Here's how the part is built. I have some questions about the finished solid (model axes, mm). A direction names the side the tool comes from. Round coordinates to 2 decimals unless told otherwise and drop trailing zeros. Loops run counter-clockwise (first coordinate to the right, second up) from the corner with the lowest first, then second, coordinate; pieces in that order, holes last. Notation, with made-up numbers: (-2, 6.25) -> (21, 6.25) arc R20 cw to (21, 19.25) -> close; hole circle Ø10 at (89, 65). An arc over 180 degrees is marked (long way). Use one line per item in the form item = value. Start each with the question number.
Item 1: If I drill on L1, parallel to Y at x = 35, z = -9; L2, parallel to X at y = 43.5, z = 3.5; L3, parallel to X at y = 97.5, z = -10, over which ranges is the centre line in solid material (lowest first)? Write a range as [from, to].
Item 2: Thinking about a two-plate mould opening in Z: for faces 4 (the face through (59, 11, -2)), 5 (the face through (59, 94.75, -4)), 6 (the face through (5.7, 100, -1)), 7 (the face through (60, 47, 0)), which applies, released by +Z, released by -Z, zero draft, split by the parting line, or undercut?
Item 3: If we section it at B-B (y = 86): Write out the boundary of the cut face in (x, z).
Item 4: If we section it at A-A (x = 34): Write out the boundary of the cut face in (y, z), then the cut area to 3 significant figures.
Item 5: For faces 1 (the face through (31, -3, -3)), 2 (the face through (38, 101, -7)), 3 (the face through (54.75, 99, -4)), which set-ups out of +Z, -Z, +X, -X, +Y, -Y let a thin tool reach every point of the face, with its end or its side?
Item 6: If we section it at C-C (x = 15): Write out the boundary of the cut face in (y, z), then the cut area to 3 significant figures.
Item 7: I'm going to push a flat-ended pin straight in: pin 1 Ø4 at (x, y) = (57, 7) entering from +Z. Where does the tip first touch, or does it pass through?
```python
from build123d import *

# Parameters (mm, degrees)
SKICA1_W                 = 67
SKICA1_H                 = 107
SKICA1_W_2               = 61
SKICA1_H_2               = 101
P_IDAT_VYSUNUT_M1_DEPTH  = 7
P_IDAT_VYSUNUT_M2_DEPTH  = 13
SKICA3_R                 = 1.5
ODEBRAT_VYSUNUT_M1_DEPTH = 13
ODEBRAT_START            = -4.8
ODEBRAT_VYSUNUT_M2_DEPTH = 4.8
ODEBRAT_VYSUNUT_M4_DEPTH = 123.804723036
ZAOBLIT1_R               = 3
SKICA5_W                 = 4
SKICA5_H                 = 8.5
SKICA5_H_2               = 13
P_IDAT_VYSUNUT_M3_DEPTH  = 3
ZKOSEN_1_SIZE            = 3
SKICA6_W                 = 4
SKICA6_H                 = 8.5
SKICA6_H_2               = 13
P_IDAT_VYSUNUT_M4_DEPTH  = 3
ZKOSEN_2_SIZE            = 3
SKICA7_W                 = 9.5
SKICA7_H                 = 7.5
ODEBRAT_VYSUNUT_M3_DEPTH = 10
SKICA9_W                 = 9.5
SKICA9_H                 = 1.25
P_IDAT_VYSUNUT_M5_DEPTH  = 4
ZAOBLIT2_R               = 1
SKICA10_W                = 19.3
SKICA10_H                = 2.8
ODEBRAT_VYSUNUT_M5_DEPTH = 6
SKICA11_R                = 1.5
ODEBRAT_VYSUNUT_M6_DEPTH = 4
SKICA13_R                = 2.5
P_IDAT_VYSUNUT_M6_DEPTH  = 1


with BuildPart() as part:
    # Skica1 → Přidat vysunutím1 (new body)
    with BuildSketch(Plane.XY):
        with Locations((30.5, 50.5)):
            Rectangle(SKICA1_W, SKICA1_H)
        with Locations((30.5, 50.5)):
            Rectangle(SKICA1_W_2, SKICA1_H_2, mode=Mode.SUBTRACT)
    extrude(amount=P_IDAT_VYSUNUT_M1_DEPTH)

    # Skica2 → Přidat vysunutím2 (add)
    with BuildSketch(Plane(origin=(0, 0, 0), x_dir=(-1, 0, 0), z_dir=(0, 0, -1))):
        with BuildLine():
            ThreePointArc((-53, 0), (-53.14730658, -1.5281381), (-53.583801513, -3))
            Line((-53.583801513, -3), (-7.416198487, -3))
            ThreePointArc((-7.416198487, -3), (-7.85269342, -1.5281381), (-8, 0))
            Line((-8, 0), (-53, 0))
        make_face()
        with BuildLine():
            ThreePointArc((-61, 8), (-62.5281381, 7.85269342), (-64, 7.416198487))
            Line((-64, 7.416198487), (-64, -3))
            Line((-64, -3), (-53.583801513, -3))
            ThreePointArc((-53.583801513, -3), (-53.14730658, -1.5281381), (-53, 0))
            Line((-53, 0), (-61, 0))
            Line((-61, 0), (-61, 8))
        make_face()
        with BuildLine():
            ThreePointArc((-53, 0), (-55.343145751, 5.656854249), (-61, 8))
            Line((-61, 8), (-61, 0))
            Line((-61, 0), (-53, 0))
        make_face()
        with BuildLine():
            ThreePointArc((-61, 93), (-62.5281381, 93.14730658), (-64, 93.583801513))
            Line((-64, 93.583801513), (-64, 7.416198487))
            ThreePointArc((-64, 7.416198487), (-62.5281381, 7.85269342), (-61, 8))
            Line((-61, 8), (-61, 93))
        make_face()
        with BuildLine():
            Line((-53.583801513, 104), (-64, 104))
            Line((-64, 104), (-64, 93.583801513))
            ThreePointArc((-64, 93.583801513), (-62.5281381, 93.14730658), (-61, 93))
            Line((-61, 93), (-61, 101))
            Line((-61, 101), (-53, 101))
            ThreePointArc((-53, 101), (-53.14730658, 102.5281381), (-53.583801513, 104))
        make_face()
        with BuildLine():
            ThreePointArc((-61, 93), (-55.343145751, 95.343145751), (-53, 101))
            Line((-53, 101), (-61, 101))
            Line((-61, 101), (-61, 93))
        make_face()
        with BuildLine():
            Line((-7.416198487, 104), (-53.583801513, 104))
            ThreePointArc((-53.583801513, 104), (-53.14730658, 102.5281381), (-53, 101))
            Line((-53, 101), (-8, 101))
            ThreePointArc((-8, 101), (-7.85269342, 102.5281381), (-7.416198487, 104))
        make_face()
        with BuildLine():
            Line((3, 104), (-7.416198487, 104))
            ThreePointArc((-7.416198487, 104), (-7.85269342, 102.5281381), (-8, 101))
            Line((-8, 101), (0, 101))
            Line((0, 101), (0, 93))
            ThreePointArc((0, 93), (1.5281381, 93.14730658), (3, 93.583801513))
            Line((3, 93.583801513), (3, 104))
        make_face()
        with BuildLine():
            Line((0, 101), (-8, 101))
            ThreePointArc((-8, 101), (-5.656854249, 95.343145751), (0, 93))
            Line((0, 93), (0, 101))
        make_face()
        with BuildLine():
            Line((3, 7.416198487), (3, 93.583801513))
            ThreePointArc((3, 93.583801513), (1.5281381, 93.14730658), (0, 93))
            Line((0, 93), (0, 8))
            ThreePointArc((0, 8), (1.5281381, 7.85269342), (3, 7.416198487))
        make_face()
        with BuildLine():
            Line((3, -3), (3, 7.416198487))
            ThreePointArc((3, 7.416198487), (1.5281381, 7.85269342), (0, 8))
            Line((0, 8), (0, 0))
            Line((0, 0), (-8, 0))
            ThreePointArc((-8, 0), (-7.85269342, -1.5281381), (-7.416198487, -3))
            Line((-7.416198487, -3), (3, -3))
        make_face()
        with BuildLine():
            Line((0, 0), (0, 8))
            ThreePointArc((0, 8), (-5.656854249, 5.656854249), (-8, 0))
            Line((-8, 0), (0, 0))
        make_face()
    extrude(amount=P_IDAT_VYSUNUT_M2_DEPTH)

    # Skica3 → Odebrat vysunutím1 (cut)
    with BuildSketch(Plane.XY):
        with Locations((3.5, 97.5)):
            Circle(SKICA3_R)
        with Locations((3.5, 3.5)):
            Circle(SKICA3_R)
        with Locations((57.5, 3.5)):
            Circle(SKICA3_R)
        with Locations((57.5, 97.5)):
            Circle(SKICA3_R)
    extrude(amount=-ODEBRAT_VYSUNUT_M1_DEPTH, mode=Mode.SUBTRACT)

    # Skica4 → Odebrat vysunutím2 (cut)
    with BuildSketch(Plane(origin=(0, 0, -13), x_dir=(-1, 0, 0), z_dir=(0, 0, -1)).offset(ODEBRAT_START)):
        with BuildLine():
            Line((-53, 101), (-61, 101))
            Line((-61, 101), (-61, 93))
            ThreePointArc((-61, 93), (-55.343145751, 95.343145751), (-53, 101))
        make_face()
    extrude(amount=ODEBRAT_VYSUNUT_M2_DEPTH, mode=Mode.SUBTRACT)

    # Skica8 → Odebrat vysunutím4 (cut, through all)
    with BuildSketch(Plane.XY):
        with BuildLine():
            Line((61, 94.75), (57.5, 94.75))
            ThreePointArc((57.5, 94.75), (55.555456352, 95.555456352), (54.75, 97.5))
            Line((54.75, 97.5), (54.75, 101))
            Line((54.75, 101), (53, 101))
            ThreePointArc((53, 101), (55.343145751, 95.343145751), (61, 93))
            Line((61, 93), (61, 94.75))
        make_face()
    extrude(amount=-ODEBRAT_VYSUNUT_M4_DEPTH, mode=Mode.SUBTRACT)

    # Zaoblit1
    zaoblit1_edges = [part.edges().sort_by_distance(p)[0] for p in [
        (-3, 104, -3),
        (64, 104, -3),
        (64, -3, -3),
        (-3, -3, -3),
    ]]
    fillet(zaoblit1_edges, radius=ZAOBLIT1_R)

    # Skica5 → Přidat vysunutím3 (add)
    with BuildSketch(Plane(origin=(0, 0, 0), x_dir=(0, 0, -1), z_dir=(1, 0, 0))):
        with Locations((2, 11.25)):
            Rectangle(SKICA5_W, SKICA5_H)
        with Locations((2, 47.5)):
            Rectangle(SKICA5_W, SKICA5_H_2)
    extrude(amount=P_IDAT_VYSUNUT_M3_DEPTH)

    # Zkosení1
    zkosen_1_edges = [part.edges().sort_by_distance(p)[0] for p in [
        (3, 11.458099244, -4),
        (3, 47.5, -4),
    ]]
    chamfer(zkosen_1_edges, length=ZKOSEN_1_SIZE - 0.0001)  # a hair under: the kernel refuses the full size

    # Skica6 → Přidat vysunutím4 (add)
    with BuildSketch(Plane.ZY.offset(-61)):
        with Locations((-2, 11.25)):
            Rectangle(SKICA6_W, SKICA6_H)
        with Locations((-2, 47.5)):
            Rectangle(SKICA6_W, SKICA6_H_2)
    extrude(amount=P_IDAT_VYSUNUT_M4_DEPTH)

    # Zkosení2
    zkosen_2_edges = [part.edges().sort_by_distance(p)[0] for p in [
        (58, 11.458099244, -4),
        (58, 47.5, -4),
    ]]
    chamfer(zkosen_2_edges, length=ZKOSEN_2_SIZE - 0.0001)  # a hair under: the kernel refuses the full size

    # Skica7 → Odebrat vysunutím3 (cut)
    with BuildSketch(Plane(origin=(0, 104, 0), x_dir=(1, 0, 0), z_dir=(0, 1, 0))):
        with Locations((48.75, 9.25)):
            Rectangle(SKICA7_W, SKICA7_H)
    extrude(amount=-ODEBRAT_VYSUNUT_M3_DEPTH, mode=Mode.SUBTRACT)

    # Skica9 → Přidat vysunutím5 (add)
    with BuildSketch(Plane(origin=(0, 0, -13), x_dir=(-1, 0, 0), z_dir=(0, 0, -1))):
        with Locations((-48.75, 103.375)):
            Rectangle(SKICA9_W, SKICA9_H)
    extrude(amount=-P_IDAT_VYSUNUT_M5_DEPTH)

    # Zaoblit2
    zaoblit2_edges = [part.edges().sort_by_distance(p)[0] for p in [
        (53.5, 103.375, -9),
        (44, 103.375, -9),
    ]]
    fillet(zaoblit2_edges, radius=ZAOBLIT2_R)

    # Skica10 → Odebrat vysunutím5 (cut, symmetric)
    with BuildSketch(Plane.XZ.offset(-101)):
        with Locations((15.35, -1.05)):
            Rectangle(SKICA10_W, SKICA10_H)
    extrude(amount=ODEBRAT_VYSUNUT_M5_DEPTH, both=True, mode=Mode.SUBTRACT)

    # Skica11 → Odebrat vysunutím6 (cut)
    with BuildSketch(Plane(origin=(0, 104, 0), x_dir=(1, 0, 0), z_dir=(0, 1, 0))):
        with Locations(Location((38, 7.45, 0), (0, 0, 270))):
            Circle(SKICA11_R)
        with Locations(Location((2, 7.45, 0), (0, 0, 270))):
            Circle(SKICA11_R)
    extrude(amount=-ODEBRAT_VYSUNUT_M6_DEPTH, mode=Mode.SUBTRACT)

    # Skica13 → Přidat vysunutím6 (add)
    with BuildSketch(Plane.XZ.offset(-101)):
        with Locations(Location((38, -7.45, 0), (0, 0, 270))):
            Circle(SKICA13_R)
    extrude(amount=P_IDAT_VYSUNUT_M6_DEPTH)


solid = part.part
```
Values found:
q1.L1 = [-3, 0], [101, 104]
q1.L2 = [-3, 0], [61, 64]
q1.L3 = [-3, 2], [5, 7.19], [61, 64]
q2.face_4 = released by -Z
q2.face_5 = zero draft
q2.face_6 = undercut
q2.face_7 = released by +Z
q3.outline = (-3, -13) -> (0, -13) -> (0, 7) -> (-3, 7) -> close; (61, -13) -> (64, -13) -> (64, 7) -> (61, 7) -> close
q4.outline = (-3, -13) -> (0, -13) -> (0, 7) -> (-3, 7) -> close; (101, -13) -> (104, -13) -> (104, 7) -> (101, 7) -> close
q4.area = 120 mm2
q5.face_1 = +Z, -Z, +X, -X, -Y
q5.face_2 = +Y
q5.face_3 = +Z, -Z
q6.outline = (-3, -13) -> (0, -13) -> (0, 7) -> (-3, 7) -> close; (101, -13) -> (104, -13) -> (104, -2.45) -> (101, -2.45) -> close; (101, 0.35) -> (104, 0.35) -> (104, 7) -> (101, 7) -> close
q6.area = 112 mm2
q7.pin_1 = 0
